```python
from build123d import *

# Parameters (mm, degrees)
SKETCH_1_R      = 3
EXTRUDE_1_DEPTH = 3
EXTRUDE_2_DEPTH = 3


with BuildPart() as part:
    # Sketch 1 → Extrude 1 (new, symmetric)
    with BuildSketch(Plane.XY):
        with BuildLine():
            Line((-6, 0), (-6, -6.821714583))
            ThreePointArc((-6, -6.821714583), (0.093730769, -8.421059064), (6, -6.22847127))
            Line((6, -6.22847127), (6, 0))
            ThreePointArc((6, 0), (5.671362579, 1.95848066), (4.721451168, 3.702417976))
            Line((4.721451168, 3.702417976), (5.777136763, 6.958366163))
            Line((5.777136763, 6.958366163), (8.152285112, 7.41624395))
            Line((8.152285112, 7.41624395), (8.152285112, 8.689000591))
            Line((8.152285112, 8.689000591), (-1.404354977, 9.690365056))
            Line((-1.404354977, 9.690365056), (-1.820682976, 5.7170896))
            ThreePointArc((-1.820682976, 5.7170896), (-4.843763922, 3.54089693), (-6, 0))
        make_face()
        Circle(SKETCH_1_R, mode=Mode.SUBTRACT)
    extrude(amount=EXTRUDE_1_DEPTH, both=True)

    # Sketch 1_4 → Extrude 2 (add, symmetric)
    with BuildSketch(Plane.XY):
        with BuildLine():
            ThreePointArc((6, -6.22847127), (3.220497082, -7.778565282), (0.10340711, -8.420576201))
            ThreePointArc((0.10340711, -8.420576201), (6.795906325, -16.266900398), (8.894248996, -26.363994395))
            ThreePointArc((8.894248996, -26.363994395), (9.133835845, -29.413676999), (12.091934084, -30.193177258))
            ThreePointArc((12.091934084, -30.193177258), (15.547503566, -26.096056877), (15.192388226, -20.748043324))
            ThreePointArc((15.192388226, -20.748043324), (11.428197085, -12.961513513), (6, -6.22847127))
        make_face()
    extrude(amount=EXTRUDE_2_DEPTH, both=True)


solid = part.part
```
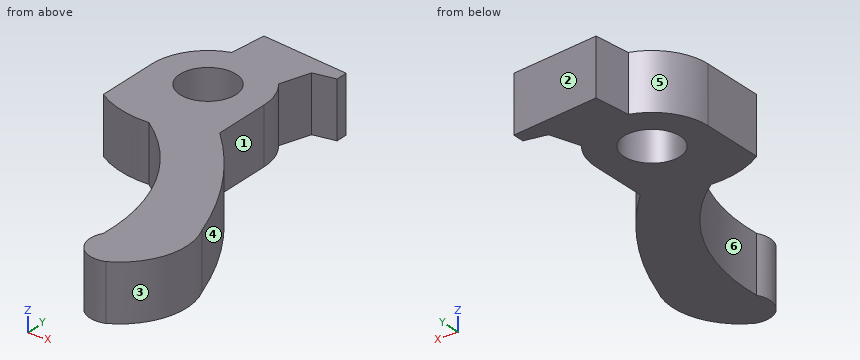
Geometry: final body of the model. Coordinates: model frame, mm. Face numbers are marked on the shaded views. A direction names the side the tool comes from. Coordinates: 2 decimals unless noted, no trailing zeros. Write each loop counter-clockwise with the first axis right and the second up, starting at its lowest first coordinate (ties: lowest second). Pieces come first, ordered by that corner, then holes. Notation, with made-up numbers: M 38,-25.5 L 90,-25.5 A20 cw 90,-8.5 Z; hole C 8.5,39.25 d3. An arc over 180 degrees is marked long. Use CSV: the item, a comma, the result in double quotes. Start each with the question number.
1. Ray query, probe 1 along Y at (x, z) = (0, 0.3); probe 2 along X at (y, z) = (-2.5, -0.7); probe 3 along Y at (x, z) = (1, -0.5). Return the intervals inside material, ascending.
2. First-contact query: P1, Ø1.4, axis at y = 8, z = -1, coming from the +X side; P2, Ø3, axis at y = -26, z = 1, coming from the +X side; P3, Ø1.5, axis at y = 5.5, z = -2, coming from the -X side; P4, Ø8, axis at x = 8, y = 2, coming from the -Z side. Flat tips, straight axial feed; report the tip coordinate or a pass-through.
3. Cut plane B-B on z = -0.8. Return the cut outline in (x, y).
4. Mould query, pull axis Y, two halves, no side actions, for the marked faces 1, 2 and 3. Classes: pulls with the +Y half, pulls with the -Y half, needs draft (parallel to the pull), parting line crosses it, or undercut.
5. Cut plane D-D on x = -4.5. Return the cut outline in (y, z), plus the area to 3 significant figures.
6. Cut plane C-C on x = 7.25. Return the cut outline in (y, z).
7. Cut plane A-A on y = 0.5. Return the cut outline in (x, z).
8. Reachability of the marked faces 4, 5 and 6 from +Z, -Z, +X, -X, +Y, -Y: full face, straight path, thin tool, end or side. Return the list, or none.
Entries:
1,probe 1,"-8.43 to -3, 3 to 9.54"
1,probe 2,"-6 to -1.66, 1.66 to 6"
1,probe 3,"-9.09 to -2.83, 2.83 to 9.44"
2,P1,"x = 8.15"
2,P2,"x = 15.88"
2,P3,"x = -3.67"
2,P4,"z = -3"
3,outline,"M -6,-6.82 A10.45 ccw 0.1,-8.42 A20.79 cw 8.89,-26.36 A2.64 ccw 12.09,-30.19 A7.16 ccw 15.19,-20.75 A37.98 ccw 6,-6.23 L 6,0 A6 ccw 4.72,3.7 L 5.78,6.96 L 8.15,7.42 L 8.15,8.69 L -1.4,9.69 L -1.82,5.72 A6 ccw -6,0 Z; hole C 0,0 d6"
4,face 1,"undercut"
4,face 2,"pulls with the +Y half"
4,face 3,"parting line crosses it"
5,outline,"M -7.61,-3 L 3.97,-3 L 3.97,3 L -7.61,3 Z"
5,area,"69.4 mm²"
6,outline,"M -17.26,-3 L -7.52,-3 L -7.52,3 L -17.26,3 Z; M 7.24,-3 L 8.78,-3 L 8.78,3 L 7.24,3 Z"
7,outline,"M -5.98,-3 L -2.96,-3 L -2.96,3 L -5.98,3 Z; M 2.96,-3 L 5.98,-3 L 5.98,3 L 2.96,3 Z"
8,face 4,"+Z, -Z, +X"
8,face 5,"+Z, -Z, -X, +Y"
8,face 6,"+Z, -Z, -X"
